Geometry: final body of the model. Coordinates: model frame, mm. Face numbers are marked on the shaded views. A direction names the side the tool comes from. Give positions to 0.01 mm unless a question says otherwise; leave off trailing zeros. Order: outer loops, then holes, each group sorted by start corner. A loop starts at its lowest first (then second) coordinate and runs counter-clockwise, first axis right, second up. Notation, with made-up numbers: (-15.5, -17) -> (12.5, -17) arc R17 cw to (12.5, -8) -> close; hole circle Ø9 at (55.25, 17). An arc over 180 degrees is marked (long way). Write item = value, one per line.
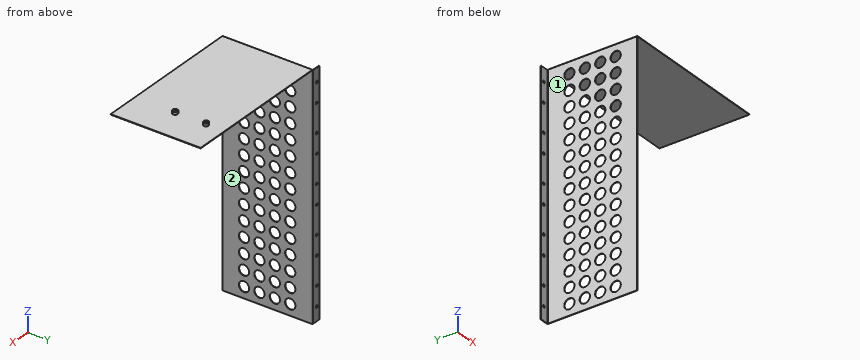
```python
from build123d import *

# Parameters (mm, degrees)
SKETCH1_W                    = 298
SKETCH1_H                    = 175
BASE_FLANGE1_DEPTH           = 1
EDGE_FLANGE1_STRIP_W         = 5.4732
EDGE_FLANGE1_STRIP_H         = 1
EDGE_FLANGE1_STRIP_CUT_DEPTH = 175
EDGE_FLANGE1_DEPTH           = 175
EDGE_FLANGE2_STRIP_W         = 5.4732
EDGE_FLANGE2_STRIP_H         = 1
EDGE_FLANGE2_STRIP_CUT_DEPTH = 463.2634
EDGE_FLANGE2_DEPTH           = 463.2634
SKETCH21_R                   = 5
SKETCH21_R_2                 = 3
BOSS_EXTRUDE2_DEPTH          = 5
SKETCH22_R                   = 10
CUT_EXTRUDE1_DEPTH           = 10
SKETCH24_R                   = 2.5
CUT_EXTRUDE2_DEPTH           = 1


# Sheet-metal steps are written as plain solids
with BuildPart() as part:
    # Sketch1 → Base-Flange1 (new body)
    with BuildSketch(Plane.XY):
        Rectangle(SKETCH1_W, SKETCH1_H)
    extrude(amount=-BASE_FLANGE1_DEPTH)

    # Edge-Flange1 strip (across the edge) → Edge-Flange1 strip cut (cut)
    with BuildSketch(Plane(origin=(-149, -87.5, -1), x_dir=(1, 0, 0), z_dir=(0, 1, 0))):
        with Locations((-1, -0.5)):
            Rectangle(EDGE_FLANGE1_STRIP_W, EDGE_FLANGE1_STRIP_H)
    extrude(amount=EDGE_FLANGE1_STRIP_CUT_DEPTH, mode=Mode.SUBTRACT)

    # Edge-Flange1 section (across the edge) → Edge-Flange1 (add)
    with BuildSketch(Plane(origin=(-149, -87.5, -1), x_dir=(1, 0, 0), z_dir=(0, 1, 0))):
        with BuildLine():
            Line((0, 0.7366), (0, 464))
            Line((0, 464), (1, 464))
            Line((1, 464), (1, 0.7366))
            ThreePointArc((1, 0.7366), (1.215745145, 0.215745145), (1.7366, 0))
            Line((1.7366, 0), (1.7366, -1))
            ThreePointArc((1.7366, -1), (0.508638364, -0.491361636), (0, 0.7366))
        make_face()
    extrude(amount=EDGE_FLANGE1_DEPTH)

    # Edge-Flange2 strip (across the edge) → Edge-Flange2 strip cut (cut)
    with BuildSketch(Plane(origin=(-149, 87.5, -1.7366), x_dir=(0, -1, 0), z_dir=(0, 0, -1))):
        with Locations((-1, -0.5)):
            Rectangle(EDGE_FLANGE2_STRIP_W, EDGE_FLANGE2_STRIP_H)
    extrude(amount=EDGE_FLANGE2_STRIP_CUT_DEPTH, mode=Mode.SUBTRACT)

    # Edge-Flange2 section (across the edge) → Edge-Flange2 (add)
    with BuildSketch(Plane(origin=(-149, 87.5, -1.7366), x_dir=(0, -1, 0), z_dir=(0, 0, -1))):
        with BuildLine():
            Line((0, 0.7366), (0, 17))
            Line((0, 17), (1, 17))
            Line((1, 17), (1, 0.7366))
            ThreePointArc((1, 0.7366), (1.215745145, 0.215745145), (1.7366, 0))
            Line((1.7366, 0), (1.7366, -1))
            ThreePointArc((1.7366, -1), (0.508638364, -0.491361636), (0, 0.7366))
        make_face()
    extrude(amount=EDGE_FLANGE2_DEPTH)

    # Sketch21 → Boss-Extrude2 (add)
    # profile 1 of 2: a face of its own
    with BuildSketch(Plane.XY):
        with Locations(Location((87, 52.5, 0), (0, 0, 180))):
            Circle(SKETCH21_R)
        with Locations((87, 52.5)):
            Circle(SKETCH21_R_2, mode=Mode.SUBTRACT)
    # profile 2 of 2: a face of its own
    with BuildSketch(Plane.XY):
        with Locations(Location((87, -7.5, 0), (0, 0, 180))):
            Circle(SKETCH21_R)
        with Locations((87, -7.5)):
            Circle(SKETCH21_R_2, mode=Mode.SUBTRACT)
    extrude(amount=BOSS_EXTRUDE2_DEPTH)

    # Sketch22 → Cut-Extrude1 (cut)
    with BuildSketch(Plane.ZY.offset(149)):
        with Locations((-443.375, 44.1334)):
            Circle(SKETCH22_R)
        with Locations((-413.375, 44.1334)):
            Circle(SKETCH22_R)
        with Locations((-383.375, 44.1334)):
            Circle(SKETCH22_R)
        with Locations((-353.375, 44.1334)):
            Circle(SKETCH22_R)
        with Locations((-323.375, 44.1334)):
            Circle(SKETCH22_R)
        with Locations((-293.375, 44.1334)):
            Circle(SKETCH22_R)
        with Locations((-263.375, 44.1334)):
            Circle(SKETCH22_R)
        with Locations((-233.375, 44.1334)):
            Circle(SKETCH22_R)
        with Locations((-203.375, 44.1334)):
            Circle(SKETCH22_R)
        with Locations((-173.375, 44.1334)):
            Circle(SKETCH22_R)
        with Locations((-143.375, 44.1334)):
            Circle(SKETCH22_R)
        with Locations((-113.375, 44.1334)):
            Circle(SKETCH22_R)
        with Locations((-83.375, 44.1334)):
            Circle(SKETCH22_R)
        with Locations((-413.375, 14.1334)):
            Circle(SKETCH22_R)
        with Locations((-383.375, 14.1334)):
            Circle(SKETCH22_R)
        with Locations((-353.375, 14.1334)):
            Circle(SKETCH22_R)
        with Locations((-323.375, 14.1334)):
            Circle(SKETCH22_R)
        with Locations((-293.375, 14.1334)):
            Circle(SKETCH22_R)
        with Locations((-263.375, 14.1334)):
            Circle(SKETCH22_R)
        with Locations((-233.375, 14.1334)):
            Circle(SKETCH22_R)
        with Locations((-203.375, 14.1334)):
            Circle(SKETCH22_R)
        with Locations((-173.375, 14.1334)):
            Circle(SKETCH22_R)
        with Locations((-143.375, 14.1334)):
            Circle(SKETCH22_R)
        with Locations((-113.375, 14.1334)):
            Circle(SKETCH22_R)
        with Locations((-83.375, 14.1334)):
            Circle(SKETCH22_R)
        with Locations((-413.375, -15.8666)):
            Circle(SKETCH22_R)
        with Locations((-383.375, -15.8666)):
            Circle(SKETCH22_R)
        with Locations((-353.375, -15.8666)):
            Circle(SKETCH22_R)
        with Locations((-323.375, -15.8666)):
            Circle(SKETCH22_R)
        with Locations((-293.375, -15.8666)):
            Circle(SKETCH22_R)
        with Locations((-263.375, -15.8666)):
            Circle(SKETCH22_R)
        with Locations((-233.375, -15.8666)):
            Circle(SKETCH22_R)
        with Locations((-203.375, -15.8666)):
            Circle(SKETCH22_R)
        with Locations((-173.375, -15.8666)):
            Circle(SKETCH22_R)
        with Locations((-143.375, -15.8666)):
            Circle(SKETCH22_R)
        with Locations((-113.375, -15.8666)):
            Circle(SKETCH22_R)
        with Locations((-83.375, -15.8666)):
            Circle(SKETCH22_R)
        with Locations((-413.375, -45.8666)):
            Circle(SKETCH22_R)
        with Locations((-383.375, -45.8666)):
            Circle(SKETCH22_R)
        with Locations((-353.375, -45.8666)):
            Circle(SKETCH22_R)
        with Locations((-323.375, -45.8666)):
            Circle(SKETCH22_R)
        with Locations((-293.375, -45.8666)):
            Circle(SKETCH22_R)
        with Locations((-263.375, -45.8666)):
            Circle(SKETCH22_R)
        with Locations((-233.375, -45.8666)):
            Circle(SKETCH22_R)
        with Locations((-203.375, -45.8666)):
            Circle(SKETCH22_R)
        with Locations((-173.375, -45.8666)):
            Circle(SKETCH22_R)
        with Locations((-143.375, -45.8666)):
            Circle(SKETCH22_R)
        with Locations((-113.375, -45.8666)):
            Circle(SKETCH22_R)
        with Locations((-83.375, -45.8666)):
            Circle(SKETCH22_R)
        with Locations((-443.375, 14.1334)):
            Circle(SKETCH22_R)
        with Locations((-443.375, -15.8666)):
            Circle(SKETCH22_R)
        with Locations((-443.375, -45.8666)):
            Circle(SKETCH22_R)
        with Locations((-53.375, 44.1334)):
            Circle(SKETCH22_R)
        with Locations((-23.375, 44.1334)):
            Circle(SKETCH22_R)
        with Locations((-53.375, 14.1334)):
            Circle(SKETCH22_R)
        with Locations((-23.375, 14.1334)):
            Circle(SKETCH22_R)
        with Locations((-53.375, -15.8666)):
            Circle(SKETCH22_R)
        with Locations((-23.375, -15.8666)):
            Circle(SKETCH22_R)
        with Locations((-53.375, -45.8666)):
            Circle(SKETCH22_R)
        with Locations((-23.375, -45.8666)):
            Circle(SKETCH22_R)
    extrude(amount=-CUT_EXTRUDE1_DEPTH, mode=Mode.SUBTRACT)

    # Sketch24 → Cut-Extrude2 (cut)
    with BuildSketch(Plane(origin=(0, 87.5, 0), x_dir=(1, 0, 0), z_dir=(0, 1, 0))):
        with Locations(Location((-159.25, 438, 0), (0, 0, 180))):
            Circle(SKETCH24_R)
        with Locations(Location((-159.25, 400, 0), (0, 0, 180))):
            Circle(SKETCH24_R)
        with Locations(Location((-159.25, 345, 0), (0, 0, 180))):
            Circle(SKETCH24_R)
        with Locations(Location((-159.25, 307, 0), (0, 0, 180))):
            Circle(SKETCH24_R)
        with Locations(Location((-159.25, 252, 0), (0, 0, 180))):
            Circle(SKETCH24_R)
        with Locations(Location((-159.25, 214, 0), (0, 0, 180))):
            Circle(SKETCH24_R)
        with Locations(Location((-159.25, 159, 0), (0, 0, 180))):
            Circle(SKETCH24_R)
        with Locations(Location((-159.25, 121, 0), (0, 0, 180))):
            Circle(SKETCH24_R)
        with Locations(Location((-159.25, 66, 0), (0, 0, 180))):
            Circle(SKETCH24_R)
        with Locations(Location((-159.25, 28, 0), (0, 0, 180))):
            Circle(SKETCH24_R)
    extrude(amount=-CUT_EXTRUDE2_DEPTH, mode=Mode.SUBTRACT)


solid = part.part
```
1) Section query B-B (x = 7). Output: boundary loops of the cut face in (y, z), plus the area to 3 significant figures.
Check sheet entries:
outline = (-87.5, -1) -> (87.5, -1) -> (87.5, 0) -> (-87.5, 0) -> close
area = 175 mm²
2) Reachability of the marked faces 1 and 2 from +Z, -Z, +X, -X, +Y, -Y: full face, straight path, thin tool, end or side. Return the list, or none.
Check sheet entries:
face_1 = +Z, -Z, -X, -Y
face_2 = -Z, +X, +Y, -Y
3) Section query C-C (y = -51). Count the separate pieces of the cut face and the enclosed holes in it, plus the area to 3 significant figures.
Check sheet entries:
separate_pieces = 16
enclosed_holes = 0
area = 504 mm²
4) Line query: line 1 (Z direction, x = -50, y = 5); line 2 (X direction, y = -55.5, z = -208.5); line 3 (X direction, y = 87.1, z = -400). Output: solid intervals per line, ascending. Write a range as from..to.
Check sheet entries:
line_1 = -1..0
line_2 = -149..-148
line_3 = -166..-161.75, -156.75..-148.63
5) Section query A-A (z = -79). Output: boundary loops of the cut face in (x, y), plus the area to 3 significant figures.
Check sheet entries:
outline = (-166, 86.5) -> (-149.74, 86.5) arc R0.74 cw to (-149, 85.76) -> (-149, 53.13) -> (-148, 53.13) -> (-148, 85.76) arc R1.74 ccw to (-149.74, 87.5) -> (-166, 87.5) -> close; (-149, -87.5) -> (-148, -87.5) -> (-148, -54.86) -> (-149, -54.86) -> close; (-149, -36.87) -> (-148, -36.87) -> (-148, -24.86) -> (-149, -24.86) -> close; (-149, -6.87) -> (-148, -6.87) -> (-148, 5.14) -> (-149, 5.14) -> close; (-149, 23.13) -> (-148, 23.13) -> (-148, 35.14) -> (-149, 35.14) -> close
area = 120 mm²
6) First-contact query: P1, Ø16, axis at y = -15.87, z = -53.38, coming from the +X side; P2, Ø3.5, axis at x = 87, y = -7.5, coming from the +Z side; P3, Ø1.9, axis at x = -159.5, y = 87, coming from the +Z side; P4, Ø23, axis at y = -45.87, z = -293.38, coming from the -X side. Flat tips, straight axial feed; report the tip coordinate or a pass-through.
Check sheet entries:
P1 = through
P2 = 0
P3 = -1.74
P4 = -149
